from build123d import *

# Parameters (mm, degrees)
F0_W           = 40
F0_H           = 90
F1_DEPTH       = 30
F3_DEPTH       = 20
F4_DEPTH       = 30
F5_D           = 13.2
F5_CBORE_D     = 19.25
F5_CBORE_DEPTH = 12
F6_DEPTH       = 10
F7_DEPTH       = 15


with BuildPart() as f1:
    # F0 (on Front) → F1 (new body)
    with BuildSketch(Plane.XZ):
        with BuildLine():
            Line((0, -30), (0, 0))
            Line((0, 0), (30, 30))
            Line((30, 30), (50, 30))
            ThreePointArc((50, 30), (57.0710678119, 32.9289321881), (60, 40))
            Line((60, 40), (60, 50))
            ThreePointArc((60, 50), (57.0710678119, 57.0710678119), (50, 60))
            Line((50, 60), (-40, 60))
            ThreePointArc((-40, 60), (-47.0710678119, 57.0710678119), (-50, 50))
            Line((-50, 50), (-50, -30))
            ThreePointArc((-50, -30), (-47.0710678119, -37.0710678119), (-40, -40))
            Line((-40, -40), (-10, -40))
            ThreePointArc((-10, -40), (-2.9289321881, -37.0710678119), (0, -30))
        make_face()
        with Locations((-25, 10)):
            Rectangle(F0_W, F0_H, mode=Mode.SUBTRACT)
        with Locations((-25, 10)):
            Rectangle(F0_W, F0_H)
    extrude(amount=-F1_DEPTH)

    # F2 (on face) → F3 (cut)
    with BuildSketch(Plane.XZ):
        with BuildLine():
            Line((-15, -10), (-15, 30))
            ThreePointArc((-15, 30), (-25, 40), (-35, 30))
            Line((-35, 30), (-35, -10))
            ThreePointArc((-35, -10), (-25, -20), (-15, -10))
        make_face()
        with BuildLine():
            ThreePointArc((-30, 30), (-25, 35), (-20, 30))
            Line((-20, 30), (-20, -10))
            ThreePointArc((-20, -10), (-25, -15), (-30, -10))
            Line((-30, -10), (-30, 30))
        make_face(mode=Mode.SUBTRACT)
    extrude(amount=-F3_DEPTH, mode=Mode.SUBTRACT)

    # F2 (on face) → F4 (cut)
    with BuildSketch(Plane.XZ):
        with BuildLine():
            Line((-20, -10), (-20, 30))
            ThreePointArc((-20, 30), (-25, 35), (-30, 30))
            Line((-30, 30), (-30, -10))
            ThreePointArc((-30, -10), (-25, -15), (-20, -10))
        make_face()
    extrude(amount=-F4_DEPTH, mode=Mode.SUBTRACT)

    # F5 (through all)
    with Locations(Plane.XZ):
        with Locations((45, 45)):
            CounterBoreHole(F5_D / 2, F5_CBORE_D / 2, F5_CBORE_DEPTH)

    # F2 (on face) → F6 (cut)
    with BuildSketch(Plane.XZ):
        with BuildLine():
            ThreePointArc((-35, 55), (-42.0710678119, 52.0710678119), (-45, 45))
            Line((-45, 45), (-45, -25))
            ThreePointArc((-45, -25), (-42.0710678119, -32.0710678119), (-35, -35))
            Line((-35, -35), (-15, -35))
            ThreePointArc((-15, -35), (-7.9289321881, -32.0710678119), (-5, -25))
            Line((-5, -25), (-5, 45))
            ThreePointArc((-5, 45), (-7.9289321881, 52.0710678119), (-15, 55))
            Line((-15, 55), (-35, 55))
        make_face()
        with BuildLine():
            Line((-30.0000007451, 50.0000007451), (-19.9999992549, 50.0000007451))
            ThreePointArc((-19.9999992549, 50.0000007451), (-12.9289314431, 47.0710685569), (-9.9999992549, 40.0000007451))
            Line((-9.9999992549, 40.0000007451), (-9.9999992549, -20.0000007451))
            ThreePointArc((-9.9999992549, -20.0000007451), (-12.9289314431, -27.0710685569), (-19.9999992549, -30.0000007451))
            Line((-19.9999992549, -30.0000007451), (-30.0000007451, -30.0000007451))
            ThreePointArc((-30.0000007451, -30.0000007451), (-37.0710685569, -27.0710685569), (-40.0000007451, -20.0000007451))
            Line((-40.0000007451, -20.0000007451), (-40.0000007451, 40.0000007451))
            ThreePointArc((-40.0000007451, 40.0000007451), (-37.0710685569, 47.0710685569), (-30.0000007451, 50.0000007451))
        make_face(mode=Mode.SUBTRACT)
    extrude(amount=-F6_DEPTH, mode=Mode.SUBTRACT)

    # F7 (cut): a face of the model
    f7_faces = [f1.faces().sort_by_distance(p)[0] for p in [
        (-36.4669162447, 0, -26.4669162447),
    ]]
    extrude(f7_faces, amount=-F7_DEPTH, mode=Mode.SUBTRACT)


solid = f1.part
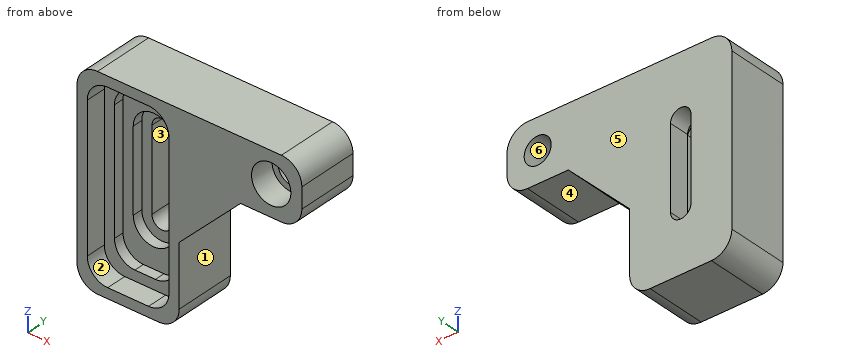
For this review, take the finished solid that the model builds, in its own axes (mm). Face numbers are marked on the shaded views. A direction names the side the tool comes from. Round coordinates to 2 decimals unless told otherwise and drop trailing zeros. Loops run counter-clockwise (first coordinate to the right, second up) from the corner with the lowest first, then second, coordinate; pieces in that order, holes last. Notation, with made-up numbers: (-5.5, 0) - (1.5, 0) arc R33 ccw to (1.5, 35) - close; hole circle Ø6 at (-21, 13.5). An arc over 180 degrees is marked (long way). One line per item, written item: value. Start each with the question number.
Item 1: For L1, parallel to Z at x = -32.5, y = 9.5; L2, parallel to Z at x = 45, y = 20; L3, parallel to Y at x = -38, z = 37.5, list the stretches that pass through material, from the lowest coordinate up.
Item 2: Take a section at C-C (y = 28.25). Give the boundary of the cut face in (x, z), plus the area to 3 significant figures.
Item 3: Take a section at A-A (z = 12.5). Give the boundary of the cut face in (x, y), plus the area to 4 significant figures.
Item 4: For the marked faces 1, 2 and 3, list the 3-axis set-ups (+Z, -Z, +X, -X, +Y, -Y) from which the entire face can be reached by the end or side of a thin tool; tool diameter is ignored.
Item 5: Clearance check with flat-ended pins moving along their axes: pin 1 Ø3 at (y, z) = (7, -12.5) entering from +X; pin 2 Ø2 at (x, z) = (-22.5, 14) entering from -Y; pin 3 Ø8 at (y, z) = (5.5, 18.5) entering from +X; pin 4 Ø16 at (x, y) = (42.5, 9) entering from -Z. State where each tip first meets the part, or that it passes through.
Item 6: The part is to be moulded in two halves that separate along Z. For the marked faces 4, 5 and 6, say which applies: +Z half, -Z half, draft (parallel to the pull), parting line (faces both ways), or undercut.
Item 7: Take a section at D-D (x = 45). Give the boundary of the cut face in (y, z) (3 decimals), plus the area to 3 significant figures.
Item 8: Take a section at B-B (x = -25). Give the boundary of the cut face in (y, z).
Answer below:
1. L1: z = -40 to -35, 55 to 60
1. L2: z = 30 to 38.4, 51.6 to 60
1. L3: y = 15 to 30
2. outline: (-50, -30) arc R10 ccw to (-40, -40) - (-10, -40) arc R10 ccw to (0, -30) - (0, 0) - (30, 30) - (50, 30) arc R10 ccw to (60, 40) - (60, 50) arc R10 ccw to (50, 60) - (-40, 60) arc R10 ccw to (-50, 50) - close; hole (-30, -10) arc R5 ccw to (-20, -10) - (-20, 30) arc R5 ccw to (-30, 30) - close; hole circle Ø13.2 at (45, 45)
2. area: 6,530 mm2
3. outline: (-50, 0) - (-45, 0) - (-45, 10) - (-40, 10) - (-40, 15) - (-35, 15) - (-35, 20) - (-30, 20) - (-30, 30) - (-50, 30) - close; (-20, 20) - (-15, 20) - (-15, 15) - (-10, 15) - (-10, 10) - (-5, 10) - (-5, 0) - (12.5, 0) - (12.5, 30) - (-20, 30) - close
3. area: 1,125 mm2
4. face 1: -Z, +X, +Y, -Y
4. face 2: -Y
4. face 3: +Y, -Y
5. pin 1: stops at x = 0
5. pin 2: passes through
5. pin 3: stops at x = 22.5
5. pin 4: stops at z = 30
6. face 4: -Z half
6. face 5: draft
6. face 6: undercut
7. outline: (0, 30) - (30, 30) - (30, 38.4) - (12, 38.4) - (12, 35.375) - (0, 35.375) - close; (0, 54.625) - (12, 54.625) - (12, 51.6) - (30, 51.6) - (30, 60) - (0, 60) - close
7. area: 431 mm2
8. outline: (0, -40) - (30, -40) - (30, -15) - (20, -15) - (20, -20) - (15, -20) - (15, -30) - (10, -30) - (10, -35) - (0, -35) - close; (0, 55) - (10, 55) - (10, 50) - (15, 50) - (15, 40) - (20, 40) - (20, 35) - (30, 35) - (30, 60) - (0, 60) - close
